CAD build for the part. Positions are in the model's coordinates, mm. A direction names the side the tool comes from. Round coordinates to 2 decimals unless told otherwise and drop trailing zeros. Write each loop counter-clockwise with the first axis right and the second up, starting at its lowest first coordinate (ties: lowest second). Pieces come first, ordered by that corner, then holes. Notation, with made-up numbers: (-33, -8) -> (-21, -8) arc R33 ccw to (-21, 20) -> close; hole circle Ø3 at (-23.5, 73.25). An arc over 180 degrees is marked (long way). Put each result on its own line as item: value. Start each with the question number.
1. Saw through at C-C on x = 22. List the corners of the cut face in (y, z).
2. 3-axis set-ups, long thin cutter, end or side, ignore diameter. For faces 1 (the flat face through (-16.4, -4.1, 21.59)), 2 (the flat face through (-35.774, -4, 11)): which of +Z, -Z, +X, -X, +Y, -Y reach the whole face in a straight line?
3. Flat gauge pin, fed straight in: P1, Ø3, axis at x = -1.5, z = 37, coming from the -Y side. Where does the tip first touch, or does it go through?
4. Drill centre lines: line 1 (Z direction, x = -5.5, y = -30); line 2 (X direction, y = -3, z = 26); line 3 (Z direction, x = 8.5, y = 4). Where is each one in solid material? Low to high. Write a range as from..to.
5. Saw through at D-D on y = -19.5. List the corners of the cut face in (x, z), and give its area (3 significant figures).
6. Saw through at B-B on x = -15.5. List the corners of the cut face in (y, z).
7. Saw through at A-A on y = -11. List the corners of the cut face in (x, z).
from build123d import *

# Parameters (mm, degrees)
F1_DEPTH = 50.8
F2_DEPTH = 21.59
F4_DEPTH = 79.241672


with BuildPart() as f1:
    # F0 (on Top) → F1 (new body)
    with BuildSketch(Plane.XY):
        with BuildLine():
            ThreePointArc((0, -16.728577), (11.82889, -11.82889), (16.728577, 0))
            ThreePointArc((16.728577, 0), (11.82889, 11.82889), (0, 16.728577))
            Line((0, 16.728577), (0, -16.728577))
        make_face()
        with BuildLine():
            Line((0, -16.728577), (0, 16.728577))
            ThreePointArc((0, 16.728577), (-16.728577, 0), (0, -16.728577))
        make_face()
    extrude(amount=F1_DEPTH)

    # F0 (on Top) → F2 (join)
    with BuildSketch(Plane.XY):
        with BuildLine():
            ThreePointArc((0, -16.728577), (-16.728577, 0), (0, 16.728577))
            Line((0, 16.728577), (0, 35.004374))
            Line((0, 35.004374), (-35.773702, 35.004374))
            Line((-35.773702, 35.004374), (-35.773702, -44.236299))
            Line((-35.773702, -44.236299), (0, -44.236299))
            Line((0, -44.236299), (0, -16.728577))
        make_face()
        with BuildLine():
            ThreePointArc((0, 16.728577), (11.82889, 11.82889), (16.728577, 0))
            ThreePointArc((16.728577, 0), (11.82889, -11.82889), (0, -16.728577))
            Line((0, -16.728577), (0, -44.236299))
            Line((0, -44.236299), (35.773702, -44.236299))
            Line((35.773702, -44.236299), (35.773702, 35.004374))
            Line((35.773702, 35.004374), (0, 35.004374))
            Line((0, 35.004374), (0, 16.728577))
        make_face()
    extrude(amount=F2_DEPTH)

    # F3 (on face) → F4 (cut, through all)
    with BuildSketch(Plane.XZ.offset(44.236299)):
        Polygon((16.728577, 50.8), (-16.728577, 50.8), (16.728577, 25.4), align=None)
    extrude(amount=-F4_DEPTH, mode=Mode.SUBTRACT)


solid = f1.part
Return value:
1. outline: (-44.24, 0) -> (35, 0) -> (35, 21.59) -> (-44.24, 21.59) -> close
2. face 1: +Z
2. face 2: +Z, -Z, -X, +Y, -Y
3. P1: stops at y = -16.73
4. line 1: z = 0..21.59
4. line 2: x = -16.46..15.94
4. line 3: z = 0..31.65
5. outline: (-35.77, 0) -> (35.77, 0) -> (35.77, 21.59) -> (-35.77, 21.59) -> close
5. area: 1,540 mm^2
6. outline: (-44.24, 0) -> (35, 0) -> (35, 21.59) -> (6.29, 21.59) -> (6.29, 49.87) -> (-6.29, 49.87) -> (-6.29, 21.59) -> (-44.24, 21.59) -> close
7. outline: (-35.77, 0) -> (35.77, 0) -> (35.77, 21.59) -> (12.6, 21.59) -> (12.6, 28.53) -> (-12.6, 47.67) -> (-12.6, 21.59) -> (-35.77, 21.59) -> close
